from build123d import *

# Parameters (mm, degrees)
BOSS_EXTRUDE1_DEPTH      = 5
BOSS_EXTRUDE2_DEPTH      = 4
SKETCH3_W                = 3
SKETCH3_H                = 47.6
BOSS_EXTRUDE3_DEPTH      = 7
SKETCH4_R                = 2.5
BOSS_EXTRUDE4_DEPTH      = 5.5
SKETCH5_R                = 3.7
CUT_EXTRUDE2_DEPTH       = 1.6
CUT_EXTRUDE4_DEPTH       = 1.6
SKETCH7_R                = 2.5
CUT_EXTRUDE6_DEPTH       = 1.6
SKETCH8_R                = 1.5
CUT_EXTRUDE8_DEPTH       = 4
M2_CLEARANCE_HOLE1_D     = 2.4
M2_CLEARANCE_HOLE1_DEPTH = 5
M2_CLEARANCE_HOLE1_TIP   = 0.721032743
M2_CLEARANCE_HOLE2_D     = 2.4
M2_CLEARANCE_HOLE2_DEPTH = 5
M2_CLEARANCE_HOLE2_TIP   = 0.721032743
M2_CLEARANCE_HOLE3_D     = 2.4
M2_CLEARANCE_HOLE3_DEPTH = 35
M2_CLEARANCE_HOLE4_D     = 2.4
M2_CLEARANCE_HOLE4_DEPTH = 35
M2_CLEARANCE_HOLE5_D     = 2.4
M2_CLEARANCE_HOLE5_DEPTH = 35
M2_CLEARANCE_HOLE6_D     = 2.4
M2_CLEARANCE_HOLE6_DEPTH = 35
FILLET1_R                = 2


with BuildPart() as part:
    # Sketch1 → Boss-Extrude1 (new body)
    with BuildSketch(Plane(origin=(0, 19.3, 0), x_dir=(1, 0, 0), z_dir=(0, 1, 0))):
        with BuildLine():
            Line((5.5, -7), (33.5, -7))
            Line((33.5, -7), (33.5, 7))
            Line((33.5, 7), (5.5, 7))
            ThreePointArc((5.5, 7), (-1.5, 0), (5.5, -7))
        make_face()
    extrude(amount=BOSS_EXTRUDE1_DEPTH)



with BuildPart() as body_2:
    # Sketch2 → Boss-Extrude2 (new body)
    with BuildSketch(Plane(origin=(0, -23.3, 0), x_dir=(1, 0, 0), z_dir=(0, 1, 0))):
        with BuildLine():
            Line((5.5, -7), (33.5, -7))
            Line((33.5, -7), (33.5, 7))
            Line((33.5, 7), (5.5, 7))
            ThreePointArc((5.5, 7), (-1.5, 0), (5.5, -7))
        make_face()
    extrude(amount=BOSS_EXTRUDE2_DEPTH)


with BuildPart() as part_1:
    add(part.part)

    add(body_2.part)  # Boss-Extrude3 merges body 2
    # Sketch3 → Boss-Extrude3 (add, symmetric)
    with BuildSketch(Plane.XY):
        with Locations((32, 0.5)):
            Rectangle(SKETCH3_W, SKETCH3_H)
    extrude(amount=BOSS_EXTRUDE3_DEPTH, both=True)

    # Sketch4 → Boss-Extrude4 (add)
    with BuildSketch(Plane(origin=(0, 24.3, 0), x_dir=(1, 0, 0), z_dir=(0, 1, 0))):
        with Locations(Location((5.5, 0, 0), (0, 0, 270))):
            Circle(SKETCH4_R)
    extrude(amount=BOSS_EXTRUDE4_DEPTH)

    # Sketch5 → Cut-Extrude2 (cut)
    with BuildSketch(Plane(origin=(0, 19.3, 0), x_dir=(1, 0, 0), z_dir=(0, 1, 0))):
        with Locations(Location((5.5, 0, 0), (0, 0, 270))):
            Circle(SKETCH5_R)
    extrude(amount=CUT_EXTRUDE2_DEPTH, mode=Mode.SUBTRACT)

    # Sketch6 → Cut-Extrude4 (cut)
    with BuildSketch(Plane(origin=(0, 19.3, 0), x_dir=(1, 0, 0), z_dir=(0, 1, 0))):
        with BuildLine():
            Line((5.5, -2.7), (20.7, -2.7))
            Line((20.7, -2.7), (20.7, 2.7))
            Line((20.7, 2.7), (5.5, 2.7))
            ThreePointArc((5.5, 2.7), (2.8, 0), (5.5, -2.7))
        make_face()
    extrude(amount=CUT_EXTRUDE4_DEPTH, mode=Mode.SUBTRACT)

    # Sketch7 → Cut-Extrude6 (cut)
    with BuildSketch(Plane(origin=(0, 20.9, 0), x_dir=(1, 0, 0), z_dir=(0, 1, 0))):
        with Locations(Location((5.5, 0, 0), (0, 0, 270))):
            Circle(SKETCH7_R)
    extrude(amount=CUT_EXTRUDE6_DEPTH, mode=Mode.SUBTRACT)

    # Sketch8 → Cut-Extrude8 (cut)
    with BuildSketch(Plane(origin=(0, -23.3, 0), x_dir=(1, 0, 0), z_dir=(0, 1, 0))):
        with Locations(Location((5.5, 0, 0), (0, 0, 270))):
            Circle(SKETCH8_R)
    extrude(amount=CUT_EXTRUDE8_DEPTH, mode=Mode.SUBTRACT)

    # M2 Clearance Hole1
    with Locations(Plane(origin=(0, 24.3, 0), x_dir=(1, 0, 0), z_dir=(0, 1, 0))):
        with Locations((15.5, 0)):
            Hole(M2_CLEARANCE_HOLE1_D / 2, depth=M2_CLEARANCE_HOLE1_DEPTH)
            with Locations((0, 0, -(M2_CLEARANCE_HOLE1_DEPTH + M2_CLEARANCE_HOLE1_TIP / 2))):  # 118° drill point
                Cone(0, M2_CLEARANCE_HOLE1_D / 2, M2_CLEARANCE_HOLE1_TIP, mode=Mode.SUBTRACT)

    # M2 Clearance Hole2
    with Locations(Plane(origin=(0, 24.3, 0), x_dir=(1, 0, 0), z_dir=(0, 1, 0))):
        with Locations((18.5, 0)):
            Hole(M2_CLEARANCE_HOLE2_D / 2, depth=M2_CLEARANCE_HOLE2_DEPTH)
            with Locations((0, 0, -(M2_CLEARANCE_HOLE2_DEPTH + M2_CLEARANCE_HOLE2_TIP / 2))):  # 118° drill point
                Cone(0, M2_CLEARANCE_HOLE2_D / 2, M2_CLEARANCE_HOLE2_TIP, mode=Mode.SUBTRACT)

    # M2 Clearance Hole3
    with Locations(Plane(origin=(33.5, 0, 0), x_dir=(0, 0, -1), z_dir=(1, 0, 0))):
        with Locations((3.5, -8)):
            Hole(M2_CLEARANCE_HOLE3_D / 2, depth=M2_CLEARANCE_HOLE3_DEPTH)

    # M2 Clearance Hole4
    with Locations(Plane(origin=(33.5, 0, 0), x_dir=(0, 0, -1), z_dir=(1, 0, 0))):
        with Locations((-3.5, -8)):
            Hole(M2_CLEARANCE_HOLE4_D / 2, depth=M2_CLEARANCE_HOLE4_DEPTH)

    # M2 Clearance Hole5
    with Locations(Plane(origin=(33.5, 0, 0), x_dir=(0, 0, -1), z_dir=(1, 0, 0))):
        with Locations((3.5, 8)):
            Hole(M2_CLEARANCE_HOLE5_D / 2, depth=M2_CLEARANCE_HOLE5_DEPTH)

    # M2 Clearance Hole6
    with Locations(Plane(origin=(33.5, 0, 0), x_dir=(0, 0, -1), z_dir=(1, 0, 0))):
        with Locations((-3.5, 8)):
            Hole(M2_CLEARANCE_HOLE6_D / 2, depth=M2_CLEARANCE_HOLE6_DEPTH)

    # Fillet1
    fillet1_edges = [part_1.edges().sort_by_distance(p)[0] for p in [
        (30.5, 19.3, 0),
        (30.5, -19.3, 0),
    ]]
    fillet(fillet1_edges, radius=FILLET1_R)


solid = part_1.part
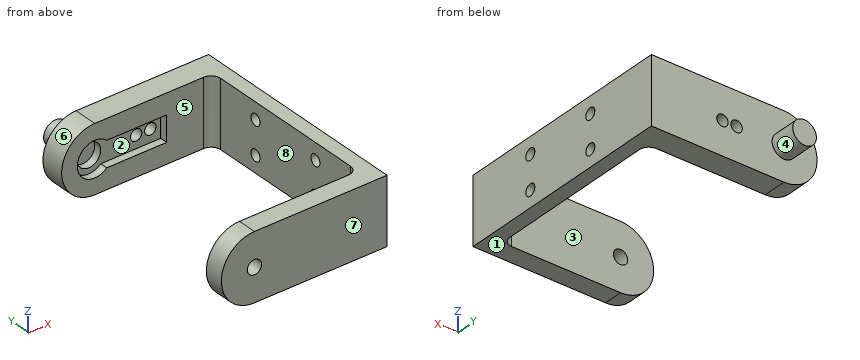
Work out the finished part from the listing and answer in its coordinate system (mm). Face numbers are marked on the shaded views. A direction names the side the tool comes from. Coordinates: 2 decimals unless noted, no trailing zeros. Loops run counter-clockwise (first coordinate to the right, second up) from the corner with the lowest first, then second, coordinate; pieces in that order, holes last. Notation, with made-up numbers: (73.5, 2) -> (103.5, 2) arc R10 cw to (103.5, 13) -> close; hole circle Ø3 at (5.5, 35.25). An arc over 180 degrees is marked (long way). Write each question's results on one line, items separated by ' | '. Start each with the question number.
1) Find section B-B on y = -8. Determine the outline of the cut face in (x, z).
2) Flat-ended cylindrical pins translate along their axes: P1, Ø4, axis at y = -8, z = -3.5, coming from the -X side; P2, Ø3, axis at x = 18.5, z = 0, coming from the +Y side; P3, Ø1.9, axis at y = 8, z = 3.5, coming from the -X side. Find the tip coordinate at first contact, or state that the pin passes through.
3) The mould has two halves that part along Y. Classify the marked faces 5, 6, 7 and 8: pulls with the +Y half, pulls with the -Y half, needs draft (parallel to the pull), parting line crosses it, or undercut.
4) Find section A-A on z = 0. Count the separate pieces of the cut face and the enclosed holes in it, then the cut area to 3 significant figures.
5) For the marked faces 1, 2, 3 and 4, determine the directions among +Z, -Z, +X, -X, +Y, -Y from which every point of the face is accessible in a straight line to the end or side of a thin tool.
6) Consider line 1 along Z through (x, y) = (5.5, 20.1); line 2 along Y through (x, z) = (11, -6); line 3 along Y through (x, z) = (12, 1.75). Determine where each line is inside the solid, lowest interval first.
7) Find section C-C on x = 15.5. Determine the outline of the cut face in (y, z).
8) Find section D-D on z = 5.5. Determine the outline of the cut face in (x, y).
Response values:
1) outline: (30.5, -7) -> (33.5, -7) -> (33.5, -4.7) -> (30.5, -4.7) -> close; (30.5, -2.3) -> (33.5, -2.3) -> (33.5, 2.3) -> (30.5, 2.3) -> close; (30.5, 4.7) -> (33.5, 4.7) -> (33.5, 7) -> (30.5, 7) -> close
2) P1: stops at x = 30.5 | P2: stops at y = 24.3 | P3: passes through
3) face 5: undercut | face 6: needs draft | face 7: pulls with the -Y half | face 8: undercut
4) separate pieces: 4 | enclosed holes: 0 | area: 393 mm^2
5) face 1: -Z, +X, -X, +Y, -Y | face 2: none | face 3: +Z, -Z, -X | face 4: +Y
6) line 1: z = -7 to -3.7, 3.7 to 7 | line 2: y = -23.3 to -19.3, 19.3 to 24.3 | line 3: y = -23.3 to -19.3, 20.9 to 24.3
7) outline: (-23.3, -7) -> (-19.3, -7) -> (-19.3, 7) -> (-23.3, 7) -> close; (19.3, -7) -> (24.3, -7) -> (24.3, -1.2) -> (20.9, -1.2) -> (20.9, -2.7) -> (19.3, -2.7) -> close; (19.3, 2.7) -> (20.9, 2.7) -> (20.9, 1.2) -> (24.3, 1.2) -> (24.3, 7) -> (19.3, 7) -> close
8) outline: (1.17, -23.3) -> (33.5, -23.3) -> (33.5, 24.3) -> (1.17, 24.3) -> (1.17, 19.3) -> (28.5, 19.3) arc R2 cw to (30.5, 17.3) -> (30.5, -17.3) arc R2 cw to (28.5, -19.3) -> (1.17, -19.3) -> close
